Autodesk Inventor part; units mm, degrees
ref_plane "YZ Plane" through (0, 0, 0) normal (1, 0, 0) x (0, 1, 0)
ref_plane "XZ Plane" through (0, 0, 0) normal (0, 1, 0) x (-1, 0, 0)
ref_plane "XY Plane" through (0, 0, 0) normal (0, 0, 1) x (1, 0, 0)
sketch "Sketch1" plane through (0, 0, 0) normal (0, 0, 1) x (1, 0, 0)
  circle A0 centre (-4.5939, 35.2781) radius 2.25
  circle A1 centre (-17.1487, 97.6266) radius 2.25
  circle A2 centre (-22.3601, 123.5071) radius 2.25
  line L0 (-4.5939, 35.2781) -> (-22.3601, 123.5071) construction
  line L1 (-0.6726, 36.0677) -> (-18.4388, 124.2967)
  line L2 (-26.2814, 122.7175) -> (-8.5151, 34.4885)
  arc A3 (-8.5151, 34.4885) -> (-0.6726, 36.0677) centre (-4.5939, 35.2781) ccw
  arc A4 (-18.4388, 124.2967) -> (-26.2814, 122.7175) centre (-22.3601, 123.5071) ccw
  point P0 (0, 0)
  point P1 (-13.477, 79.3926)
  dimension "d0" = 8
extrude "Extrusion1" add sketch "Sketch1" along normal blind 9
sketch "Sketch2" plane through (0, 0, 9) normal (0, 0, 1) x (1, 0, 0)
  circle A0 centre (-22.3601, 123.5071) radius 2.25
  circle A1 centre (-22.3601, 123.5071) radius 5
  point P0 (0, 0)
  dimension "d3" = 10
extrude "Extrusion2" cut sketch "Sketch2" against normal blind 3
fillet "Fillet1" radius 2 2 edges at (-25.6892, 119.7766, 7.5) (-17.8466, 121.3558, 7.5)
scale "Scale1" factors (0.5, 0.5, 0.5) then translate (-8.6991, 39.3015, 2.25) bodies 1
properties part number "MasiveBone1"
CAD build for the part. Positions are in the model's coordinates, mm. A direction names the side the tool comes from. Coordinates: 2 decimals unless noted, no trailing zeros. Order: outer loops, then holes, each group sorted by start corner. A loop starts at its lowest first (then second) coordinate and runs counter-clockwise, first axis right, second up.
Item 1: Two-plate mould, pull along Y, no slides. Class faces 3 (the face through (-11.24, 58.04, 4.47)), 4 (the face through (-19, 100, 5.25)), 5 (the face through (-19.36, 102.053, 3.729)), 6 (the face through (-17.46, 78.91, 4.47)): +Y half, -Y half, draft (parallel to the pull), parting line (faces both ways), or undercut.
Check sheet entries:
face 3: undercut
face 4: draft
face 5: undercut
face 6: -Y half
Item 2: Drill centre lines: L1, parallel to X at y = 88.5, z = 6.35; L2, parallel to X at y = 61, z = 3.9; L3, parallel to X at y = 85.5, z = 3.8. Where is each one in solid material? Low to high.
Check sheet entries:
L1: x = -19.39 to -18.33, -16.22 to -15.31
L2: x = -13.85 to -9.77
L3: x = -18.79 to -14.71
Item 3: 3-axis set-ups, long thin cutter, end or side, ignore diameter. For faces 1 (the face through (-15, 77, 6.75)), 2 (the face through (-17.797, 98.863, 6.01)): which of +Z, -Z, +X, -X, +Y, -Y reach the whole face in a straight line?
Check sheet entries:
face 1: +Z, +X, -X, +Y, -Y
face 2: +Z, +Y
Item 4: Band-saw the part on B-B on x = -10.75. List the corners of the cut face in (y, z).
Check sheet entries:
outline: (54.96, 2.25) - (55.84, 2.25) - (55.84, 6.75) - (54.96, 6.75) - close; (58.04, 2.25) - (65.85, 2.25) - (65.85, 6.75) - (58.04, 6.75) - close
Item 5: Band-saw the part on A-A on z = 3.8. Give the number of separate pieces and of enclosed holes in the cut face, plus the area to 3 significant figures.
Check sheet entries:
separate pieces: 1
enclosed holes: 3
area: 181 mm2
Item 6: Band-saw the part on C-C on z = 5.85. List the corners of the cut face in (x, y) (3 decimals).
Check sheet entries:
outline: (-21.178, 97.372) - (-12.957, 56.546) arc R2 ccw to (-9.035, 57.335) - (-17.256, 98.162) arc R1 ccw to (-18.706, 98.847) arc R2.5 cw to (-20.106, 98.565) arc R1 ccw to start; hole circle Ø2.25 at (-17.273, 88.115); hole circle Ø2.25 at (-10.996, 56.941)
Item 7: Band-saw the part on D-D on y = 75. List the corners of the cut face in (x, z), plus the area to 3 significant figures.
Check sheet entries:
outline: (-16.67, 2.25) - (-12.59, 2.25) - (-12.59, 6.75) - (-16.67, 6.75) - close
area: 18.4 mm2
Item 8: Pin check, flat tips, straight feed: pin 1 Ø1 at (y, z) = (64.5, 4) entering from +X; pin 2 Ø3.5 at (x, y) = (-19.88, 101.06) entering from +Z. Stop position of each tip, or through.
Check sheet entries:
pin 1: stops at x = -10.38
pin 2: stops at z = 5.25
